Could you check a few things on this model? Use its own coordinates, in mm. A direction names the side the tool comes from. Coordinates: 2 decimals unless noted, no trailing zeros. Order: outer loops, then holes, each group sorted by start corner. A loop starts at its lowest first (then second) coordinate and runs counter-clockwise, first axis right, second up.
```python
from build123d import *

# Parameters (mm, degrees)
F0_R     = 6
F1_DEPTH = 2
F2_SIZE2 = 2.5980762114
F2_SIZE  = 1.5
F4_R     = 2.5
F4_R_2   = 1.4
F5_DEPTH = 4.5
F6_R     = 1.2


# Not quite as in the source:
# - a fillet or chamfer that OpenCascade refuses, or shapes differently, is made with other operations: its cross-section is extruded or revolved along the edge and cut away or added


with BuildPart() as f1:
    # F0 (on Top) → F1 (new body)
    with BuildSketch(Plane.XY):
        Circle(F0_R)
    extrude(amount=F1_DEPTH)

    # F2
    f2_edges = [f1.edges().sort_by_distance(p)[0] for p in [
        (-6, 0, 0),
    ]]
    f2_side = f1.faces().sort_by_distance((-6, 0, 1))[0]
    chamfer(f2_edges, length=F2_SIZE, length2=F2_SIZE2, reference=f2_side)

    # F3: fillet of radius 1 on 2 edges, made by hand

    # F3_s1 → F3_t2 (revolve, cut)
    with BuildSketch(Plane.XZ):
        with BuildLine():
            ThreePointArc((3.6339745962, 0.1339745962), (3.3927936413, 0.0340741737), (3.1339745962, 0))
            Line((3.1339745962, 0), (3.4019237886, 0))
            Line((3.4019237886, 0), (3.6339745962, 0.1339745962))
        make_face()
    revolve(axis=Axis((0, 0, 0), (0, 0, 1)), mode=Mode.SUBTRACT)

    # F3_s3 → F3_t4 (revolve, cut)
    with BuildSketch(Plane.XZ):
        with BuildLine():
            ThreePointArc((6, 2), (5.8486778537, 1.5452494356), (5.5031382462, 1.2131367327))
            Line((5.5031382462, 1.2131367327), (6, 1.5))
            Line((6, 1.5), (6, 2))
        make_face()
    revolve(axis=Axis((0, 0, 1.5), (0, 0, 1)), mode=Mode.SUBTRACT)

    # F4 (on face) → F5 (join)
    with BuildSketch(Plane.XY.offset(2)):
        Circle(F4_R)
        Circle(F4_R_2, mode=Mode.SUBTRACT)
    extrude(amount=F5_DEPTH)

    # F6
    f6_edges = [f1.edges().sort_by_distance(p)[0] for p in [
        (-1.4, 0, 2),
    ]]
    fillet(f6_edges, radius=F6_R)


solid = f1.part
```
Item 1: Suppose I cut it at A-A (z = 5). List the corners of the cut face in (x, y) for me.
Item 2: For pin 1 Ø2 at (x, y) = (3.5, -2.5) entering from +Z; pin 2 Ø1 at (x, z) = (-1.5, 5) entering from +Y; pin 3 Ø2 at (y, z) = (2, 5) entering from -X, each with a flat end and sliding along its axis, tell me the tip position at first contact or that it passes through.
Item 3: Which directions (+Z, -Z, +X, -X, +Y, -Y) give clear straight access to the entire face, cutting with the end or side of a thin tool? Please do faces 1 (the face through (3, 0, 2)), 2 (the face through (1.1, -1.1, 6.5)).
Item 4: Thinking about a two-plate mould opening in X: for faces 3 (the face through (-0.54, -2.44, 4.22)), 4 (the face through (-1.4, 0.06, 4.83)), 5 (the face through (0, 0, 0)), which applies, +X half, -X half, draft (parallel to the pull), parting line (faces both ways), or undercut?
Item 5: I need wall thicknesses on line 1 (Y direction, x = 0, z = 4.95); line 2 (Z direction, x = -0.25, y = 3); line 3 (Y direction, x = 1, z = 6). Which ranges of each line are inside material? Lowest first, please.
Geometry results:
1. outline: circle Ø5 at (0, 0); hole circle Ø2.8 at (0, 0)
2. pin 1: stops at z = 2
2. pin 2: stops at y = 2.29
2. pin 3: stops at x = -2.29
3. face 1: +Z
3. face 2: +Z, +X, -X, +Y, -Y
4. face 3: parting line
4. face 4: undercut
4. face 5: draft
5. line 1: y = -2.5 to -1.4, 1.4 to 2.5
5. line 2: z = 0 to 2
5. line 3: y = -2.29 to -0.98, 0.98 to 2.29
